```python
from build123d import *

# Parameters (mm, degrees)
PAD005_DEPTH = 1.5
PAD004_DEPTH = 1.5
PAD003_DEPTH = 1.5
PAD002_DEPTH = 1.5
SKETCH001_R  = 1.5
PAD001_DEPTH = 2
SKETCH_R     = 1.5
PAD_DEPTH    = 2


with BuildPart() as body005:
    # Sketch007 (on DatumPlane) → Pad005 (new body, symmetric)
    with BuildSketch(Plane(origin=(-16.952542, -59.685824, 18.8), x_dir=(0.053778, 0.550339, 0.833207), z_dir=(-0.99526, 0.097254, 0))):
        with BuildLine():
            Line((4.207597, 37.049782), (7.231669, 35.042847))
            ThreePointArc((8.366132, 31.449048), (8.433631, 33.446315), (7.231669, 35.042847))
            Line((8.366132, 31.449048), (-0.494965, 8.82738))
            ThreePointArc((-0.494965, 8.82738), (-0.562464, 6.830114), (0.639498, 5.233582))
            Line((0.639498, 5.233582), (1.08157, 4.940199))
            Line((1.08157, 4.940199), (-1.328872, 1.308117))
            Line((-1.328872, 1.308117), (-4.396585, 3.344014))
            ThreePointArc((-5.531049, 6.937813), (-5.598548, 4.940547), (-4.396585, 3.344014))
            Line((-5.531049, 6.937813), (2.654091, 27.833816))
            ThreePointArc((2.654091, 27.833816), (2.72159, 29.831082), (1.519628, 31.427615))
            Line((1.519628, 31.427615), (0.795403, 31.908248))
            Line((0.795403, 31.908248), (4.207597, 37.049782))
        make_face()
    extrude(amount=PAD005_DEPTH, both=True)


with BuildPart() as body004:
    # Sketch006 (on DatumPlane) → Pad004 (new body, symmetric)
    with BuildSketch(Plane(origin=(39.503273, -47.519607, 18.8), x_dir=(-0.346354, 0.443537, 0.826628), z_dir=(-0.788162, -0.615468, 0))):
        with BuildLine():
            Line((0.144699, 33.044069), (4.41891, 30.134283))
            ThreePointArc((5.519197, 26.54802), (5.598713, 28.534335), (4.41891, 30.134283))
            Line((5.519197, 26.54802), (-2.355235, 6.701201))
            ThreePointArc((-2.355235, 6.701201), (-2.434751, 4.714886), (-1.254948, 3.114938))
            Line((-1.254948, 3.114938), (0.091634, 2.198216))
            Line((0.091634, 2.198216), (-2.385169, -1.439983))
            Line((-2.385169, -1.439983), (-6.306361, 1.229475))
            ThreePointArc((-7.406648, 4.815738), (-7.486164, 2.829423), (-6.306361, 1.229475))
            Line((-7.406648, 4.815738), (0.451851, 24.622399))
            ThreePointArc((0.451851, 24.622399), (0.531367, 26.608714), (-0.648436, 28.208662))
            Line((-0.648436, 28.208662), (-2.355831, 29.371017))
            Line((-2.355831, 29.371017), (0.144699, 33.044069))
        make_face()
    extrude(amount=PAD004_DEPTH, both=True)


with BuildPart() as body003:
    # Sketch005 (on DatumPlane) → Pad003 (new body, symmetric)
    with BuildSketch(Plane(origin=(41.677137, 29.657026, 18.8), x_dir=(-0.67671, -0.247278, 0.693482), z_dir=(0.343216, -0.939257, 0))):
        with BuildLine():
            Line((4.151211, 27.525873), (6.616561, 25.004493))
            ThreePointArc((7.066271, 21.401359), (7.448444, 23.27869), (6.616561, 25.004493))
            Line((7.066271, 21.401359), (0.269525, 9.689346))
            ThreePointArc((0.269525, 9.689346), (-0.112963, 7.814558), (0.715657, 6.089879))
            Line((0.715657, 6.089879), (2.232289, 4.53347))
            Line((2.232289, 4.53347), (-1.455914, 0.939527))
            Line((-1.455914, 0.939527), (-4.866698, 4.439767))
            ThreePointArc((-5.31283, 8.039234), (-5.695319, 6.164446), (-4.866698, 4.439767))
            Line((-5.31283, 8.039234), (1.04248, 18.990574))
            ThreePointArc((1.04248, 18.990574), (1.424653, 20.867905), (0.59277, 22.593708))
            Line((0.59277, 22.593708), (-0.133446, 23.336429))
            Line((-0.133446, 23.336429), (4.151211, 27.525873))
        make_face()
    extrude(amount=PAD003_DEPTH, both=True)


with BuildPart() as body002:
    # Sketch004 (on DatumPlane) → Pad002 (new body, symmetric)
    with BuildSketch(Plane(origin=(-18.553723, 55.942029, 16.8), x_dir=(0.089809, -0.501127, 0.860701), z_dir=(0.984318, 0.176404, 0))):
        with BuildLine():
            Line((1.898285, 33.961279), (5.220075, 31.912664))
            ThreePointArc((6.550331, 28.610308), (6.428026, 30.480147), (5.220075, 31.912664))
            Line((6.550331, 28.610308), (0.831685, 6.427524))
            ThreePointArc((0.831685, 6.427524), (0.901463, 4.698108), (1.914982, 3.295067))
            Line((1.914982, 3.295067), (2.353125, 2.960199))
            Line((2.353125, 2.960199), (-0.095233, -0.243246))
            Line((-0.095233, -0.243246), (-2.628776, 1.693113))
            ThreePointArc((-3.712073, 4.82557), (-3.642295, 3.096155), (-2.628776, 1.693113))
            Line((-3.712073, 4.82557), (1.549904, 25.236924))
            ThreePointArc((1.549904, 25.236924), (1.427599, 27.106762), (0.219648, 28.53928))
            Line((0.219648, 28.53928), (-0.986732, 29.283279))
            Line((-0.986732, 29.283279), (1.898285, 33.961279))
        make_face()
    extrude(amount=PAD002_DEPTH, both=True)


with BuildPart() as top:
    # Sketch001 → Pad001 (new body)
    with BuildSketch(Plane.XY.offset(18.8)):
        with BuildLine():
            Line((36.188295, 32.073721), (36.188295, -49.860845))
            ThreePointArc((33.254317, -52.860118), (35.33283, -51.958693), (36.188295, -49.860845))
            Line((-21.140977, -54.057499), (33.254317, -52.860118))
            ThreePointArc((-21.140977, -54.057499), (-28.061985, -54.235329), (-24.461971, -60.149031))
            Line((-24.461971, -60.149031), (-14.464393, -59.928959))
            Line((-14.464393, -59.928959), (-12.492298, -57.868088))
            Line((-12.492298, -57.868088), (35.620638, -56.808998))
            ThreePointArc((35.620638, -56.808998), (40.118305, -58.604702), (43.05, -54.75))
            Line((43.05, -54.75), (43.05, -44.75))
            Line((40.188295, -41.888295), (43.05, -44.75))
            Line((40.188295, 23.038295), (40.188295, -41.888295))
            Line((43.05, 25.9), (40.188295, 23.038295))
            Line((43.05, 35.9), (43.05, 25.9))
            ThreePointArc((43.05, 35.9), (40.440305, 39.650607), (36.016474, 38.507244))
            Line((-12.22825, 53.261331), (36.016474, 38.507244))
            Line((-13.817394, 56.250649), (-12.22825, 53.261331))
            Line((-23.380209, 59.175126), (-13.817394, 56.250649))
            ThreePointArc((-23.380209, 59.175126), (-28.493807, 54.681881), (-22.185612, 52.123598))
            Line((-22.185612, 52.123598), (34.395591, 34.82007))
            ThreePointArc((36.188295, 32.073721), (35.700454, 33.713555), (34.395591, 34.82007))
        make_face()
        with Locations((-24.55, 55.35)):
            Circle(SKETCH001_R, mode=Mode.SUBTRACT)
        with Locations((39.05, 35.9)):
            Circle(SKETCH001_R, mode=Mode.SUBTRACT)
        with Locations((39.05, -54.75)):
            Circle(SKETCH001_R, mode=Mode.SUBTRACT)
        with Locations((-24.55, -56.15)):
            Circle(SKETCH001_R, mode=Mode.SUBTRACT)
    extrude(amount=-PAD001_DEPTH)


with BuildPart() as fusion004:
    # Sketch → Pad (new body)
    with BuildSketch(Plane.XY):
        with BuildLine():
            Line((-15.587757, 25.048294), (15.600787, 29.714611))
            ThreePointArc((15.600787, 29.714611), (17.07661, 27.20638), (19.861672, 26.362161))
            Line((19.861672, 26.362161), (19.861672, -31.312161))
            ThreePointArc((19.861672, -31.312161), (17.312602, -31.984272), (15.735331, -34.096547))
            Line((15.735331, -34.096547), (-15.658451, -25.425119))
            ThreePointArc((-15.658451, -25.425119), (-19.612693, -20.500491), (-23.410642, -25.546635))
            Line((-23.410642, -25.546635), (-21.64152, -32.072076))
            Line((-21.64152, -32.072076), (-12.002466, -34.734526))
            Line((-12.002466, -34.734526), (-7.081864, -31.943884))
            Line((-7.081864, -31.943884), (19.55, -39.3))
            ThreePointArc((19.55, -39.3), (20.543648, -39.174618), (21.475002, -38.806332))
            Line((27.861672, -35.3), (21.475002, -38.806332))
            Line((27.861672, -25.3), (27.861672, -35.3))
            Line((23.861672, -21.3), (27.861672, -25.3))
            Line((23.861672, 16.35), (23.861672, -21.3))
            Line((27.861672, 20.35), (23.861672, 16.35))
            Line((27.861672, 30.35), (27.861672, 20.35))
            Line((21.475001, 33.856333), (27.861672, 30.35))
            ThreePointArc((21.475001, 33.856333), (20.543647, 34.224618), (19.55, 34.35))
            Line((-6.289475, 30.483992), (19.55, 34.35))
            Line((-10.83732, 33.848082), (-6.289475, 30.483992))
            Line((-20.72724, 32.368388), (-10.83732, 33.848082))
            Line((-23.267202, 25.977299), (-20.72724, 32.368388))
            ThreePointArc((-23.267202, 25.977299), (-20.030389, 20.528952), (-15.587757, 25.048294))
        make_face()
        with Locations((-19.55, 24.5)):
            Circle(SKETCH_R, mode=Mode.SUBTRACT)
        with Locations((19.55, 30.35)):
            Circle(SKETCH_R, mode=Mode.SUBTRACT)
        with Locations((19.55, -35.3)):
            Circle(SKETCH_R, mode=Mode.SUBTRACT)
        with Locations((-19.55, -24.5)):
            Circle(SKETCH_R, mode=Mode.SUBTRACT)
    extrude(amount=PAD_DEPTH)

    # Fusion: union top
    add(top.part)

    # Fusion001: union Body002
    add(body002.part)

    # Fusion002: union Body003
    add(body003.part)

    # Fusion003: union Body004
    add(body004.part)

    # Fusion004: union Body005
    add(body005.part)


solid = fusion004.part
```
Can you work these out from the model? Positions are in its coordinate system, mm. A direction names the side the tool comes from. Round coordinates to 2 decimals unless told otherwise and drop trailing zeros. Loops run counter-clockwise (first coordinate to the right, second up) from the corner with the lowest first, then second, coordinate; pieces in that order, holes last. Notation, with made-up numbers: (13.5, 37.5) -> (55.5, 37.5) arc R26 cw to (55.5, 70.5) -> close; hole circle Ø1 at (64.25, 70.25). An arc over 180 degrees is marked (long way). One line per item, written item: value. Start each with the question number.
1. If we mould it in two halves opening along Y, with no side actions, what happens to faces 5 (the flat face through (28.991, 24.999, 10.118)), 6 (the flat face through (30.34, -38.22, 10.06)), 7 (the flat face through (-18.545, 56.014, 15.26)), 8 (the cylindrical face through (19.225, 28.886, 0.986))? For each: pulls with the +Y half, pulls with the -Y half, needs draft (parallel to the pull), parting line crosses it, or undercut.
2. If we section it at A-A, the plane y = -19: Write out the boundary of the cut face in (x, z), then the cut area to 3 significant figures.
3. If we section it at B-B, the plane x = 8.5: Write out the boundary of the cut face in (y, z), then the cut area to 3 significant figures.
4. If I drill on probe 1 along Y at (x, z) = (-24.55, 17.5); probe 2 along Y at (x, z) = (19.55, 0.5); probe 3 along Y at (x, z) = (39.05, 17.35), over which ranges is the centre line in solid material (lowest first)?
5. For pin 1 (5 mm diameter, centred on x = 34, z = 5.5, fed in from +Y); pin 2 (3 mm diameter, centred on x = -20, y = -31, fed in from +Z); pin 3 (2.5 mm diameter, centred on x = -24.55, y = 55.35, fed in from -Z); pin 4 (2 mm diameter, centred on y = 2.5, z = 18, fed in from +X), each with a flat end and sliding along its axis, tell me the tip position at first contact or that it passes through.
6. For faces 1 (the flat face through (-9.58, -33.36, 0.99)), 2 (the cylindrical face through (-14.29, 32.28, 4.25)), 3 (the cylindrical face through (36.655, 27.8, 13.07)), 4 (the flat face through (41.64, 24.49, 17.81)), which set-ups out of +Z, -Z, +X, -X, +Y, -Y let a thin tool reach every point of the face, with its end or its side?
Calculated:
1. face 5: undercut
1. face 6: pulls with the -Y half
1. face 7: pulls with the +Y half
1. face 8: undercut
2. outline: (19.86, 0) -> (23.86, 0) -> (23.86, 2) -> (19.86, 2) -> close; (36.19, 16.8) -> (40.19, 16.8) -> (40.19, 18.8) -> (36.19, 18.8) -> close
2. area: 16.0 mm²
3. outline: (-57.41, 16.8) -> (-53.41, 16.8) -> (-53.41, 18.8) -> (-57.41, 18.8) -> close; (-36.25, 0) -> (-32.1, 0) -> (-32.1, 2) -> (-36.25, 2) -> close; (28.65, 0) -> (32.7, 0) -> (32.7, 2) -> (28.65, 2) -> close; (42.74, 16.8) -> (46.92, 16.8) -> (46.92, 18.8) -> (42.74, 18.8) -> close
3. area: 32.8 mm²
4. probe 1: y = -60.15 to -57.65, -54.65 to -52.15, 51.35 to 53.85, 56.85 to 59.35
4. probe 2: y = -39.3 to -36.8, -33.8 to -31.3, 26.35 to 28.85, 31.85 to 34.35
4. probe 3: y = -58.75 to -56.25, -53.25 to 34.4, 37.4 to 39.9
5. pin 1: stops at y = 28.73
5. pin 2: stops at z = 2
5. pin 3: passes through
5. pin 4: stops at x = 40.19
6. face 1: +Z, -Z, -Y
6. face 2: -X, +Y
6. face 3: -X
6. face 4: +Z, -Z, +X
